CAD build for the part. Positions are in the model's coordinates, mm. Face numbers are marked on the shaded views. A direction names the side the tool comes from. Give positions to 0.01 mm unless a question says otherwise; leave off trailing zeros. Write each loop counter-clockwise with the first axis right and the second up, starting at its lowest first coordinate (ties: lowest second). Pieces come first, ordered by that corner, then holes. Notation, with made-up numbers: (-28, -33) - (1, -33) arc R17 ccw to (1, -15) - close; hole circle Ø11 at (-4.5, 60.5). An arc over 180 degrees is marked (long way). Answer as a JSON object with one key per item and string values.
from build123d import *

# Parameters (mm, degrees)
F1_DEPTH = 25.4
F2_SIZE  = 2.54
F3_SIZE  = 2.54
F4_T     = -1.27
F6_DEPTH = 38.1
F7_R     = 1.8028918562
F7_R_2   = 1.1064766703
F7_R_3   = 1.1353765366
F7_R_4   = 1.2323804773
F7_R_5   = 1.153275907
F8_DEPTH = 12.7


with BuildPart() as f1:
    # F0 (on Front) → F1 (new body)
    with BuildSketch(Plane.XZ):
        Polygon((44.08133775, 31.9471210241), (-47.1148937941, 31.9471210241), (-47.1148937941, -27.9655810446), (-25.1216236502, -27.9655810446), (-25.1216236502, -4.8347273842), (44.08133775, -4.8347273842), (44.08133775, 7.8682824969), (-25.1216236502, 7.8682824969), (-25.1216236502, 19.2441120744), (44.08133775, 19.2441120744), align=None)
    extrude(amount=F1_DEPTH)

    # F2
    f2_edges = [f1.edges().sort_by_distance(p)[0] for p in [
        (-1.516778, -25.4, 31.947121),
    ]]
    chamfer(f2_edges, length=F2_SIZE)

    # F3
    f3_edges = [f1.edges().sort_by_distance(p)[0] for p in [
        (44.081338, -25.4, 24.325617),
        (9.479857, -25.4, 19.244112),
        (-25.121624, -25.4, 13.556197),
        (9.479857, -25.4, 7.868282),
        (44.081338, -25.4, 1.516778),
        (9.479857, -25.4, -4.834727),
        (-25.121624, -25.4, -16.400154),
        (-36.118259, -25.4, -27.965581),
        (-47.114894, -25.4, 0.72077),
    ]]
    chamfer(f3_edges, length=F3_SIZE)

    # F4
    f4_openings = [f1.faces().sort_by_distance(p)[0] for p in [
        (-1.516778, 0, 30.855962),
    ]]
    offset(amount=F4_T, openings=f4_openings, kind=Kind.INTERSECTION)

    # F5 (on face) → F6 (cut, symmetric)
    with BuildSketch(Plane(origin=(0, 0, -4.8347273842), x_dir=(1, 0, 0), z_dir=(0, 0, -1))):
        with BuildLine():
            Line((44.08133775, 0), (44.08133775, 10.256701149))
            ThreePointArc((44.08133775, 10.256701149), (-1.820328138, 7.8273301251), (-47.1148937941, 0))
            Line((-47.1148937941, 0), (44.08133775, 0))
        make_face()
    extrude(amount=F6_DEPTH, both=True, mode=Mode.SUBTRACT)

    # F7 (on face) → F8 (join)
    with BuildSketch(Plane(origin=(0, -24.13, 0), x_dir=(-1, 0, 0), z_dir=(0, 1, 0))):
        with Locations((-36.7269202571, 25.4060197622)):
            Circle(F7_R)
        with Locations((-36.7269202571, 25.4060197622)):
            Circle(F7_R_2, mode=Mode.SUBTRACT)
        with Locations((0, 25.4060197622)):
            Circle(F7_R)
        with Locations((0, 25.4060197622)):
            Circle(F7_R_3, mode=Mode.SUBTRACT)
        with Locations((36.6482846439, 25.1216236502)):
            Circle(F7_R)
        with Locations((36.6482846439, 25.1216236502)):
            Circle(F7_R_4, mode=Mode.SUBTRACT)
        with Locations((36.6482846439, -20.2868953347)):
            Circle(F7_R)
        with Locations((36.6482846439, -20.2868953347)):
            Circle(F7_R_5, mode=Mode.SUBTRACT)
    extrude(amount=F8_DEPTH)


solid = f1.part
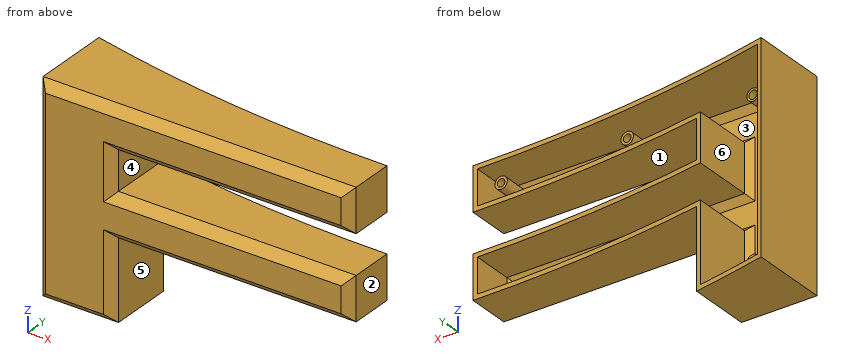
(1) Saw through at D-D, the plane x = -32.5. Give the cut face in (y, z), and give its area (3 significant figures).
Answer key:
{"outline": "(-25.4, -25.43) - (-22.86, -27.97) - (-3.13, -27.97) - (-3.13, -26.7) - (-22.33, -26.7) - (-24.13, -24.9) - (-24.13, 28.88) - (-22.33, 30.68) - (-3.13, 30.68) - (-3.13, 31.95) - (-22.86, 31.95) - (-25.4, 29.41) - close", "area": "126 mm²"}
(2) Saw through at A-A, the plane y = -20. State how many separate pieces and enclosed holes the cut face has, and give its area (3 significant figures).
Answer key:
{"separate pieces": "5", "enclosed holes": "5", "area": "577 mm²"}
(3) Saw through at B-B, the plane z = 2. Give the cut face in (x, y).
Answer key:
{"outline": "(-47.11, -22.86) - (-44.57, -25.4) - (41.54, -25.4) - (44.08, -22.86) - (44.08, -10.26) arc R388.97 cw to (42.81, -10.26) - (42.81, -22.33) - (41.02, -24.13) - (-44.05, -24.13) - (-45.84, -22.33) - (-45.84, -0.3) arc R388.97 cw to (-47.11, 0) - close"}
(4) Pull direction X, two halves, no side cores. Call the marked faces 1, 2 and 3: pulls with the +X half, pulls with the -X half, needs draft (parallel to the pull), parting line crosses it, or undercut.
Answer key:
{"face 1": "needs draft", "face 2": "pulls with the +X half", "face 3": "undercut"}
(5) Probe L1, parallel to Z at x = 0, y = -21; L2, parallel to Z at x = -21, y = -9; L3, parallel to X at y = -20.5, z = -6.5. List the from-to ranges inside material, lowest first. Write a range as [from, to].
Answer key:
{"L1": "z = [-4.83, -3.56], [6.6, 7.87], [19.24, 20.51], [23.6, 24.27], [26.54, 27.21], [30.68, 31.95]", "L2": "z = [-4.83, -3.56], [6.6, 7.87], [19.24, 20.51], [30.68, 31.95]", "L3": "x = [-47.11, -45.84], [-26.39, -25.12]"}
(6) Flat gauge pins, fed straight in: P1, Ø12, axis at x = 14, z = 11.5, coming from the -Y side; P2, Ø1, axis at x = -10, y = -7, coming from the -Z side; P3, Ø6, axis at x = -31.5, z = -19.5, coming from the +Y side. Where does each tip first touch, or does it go through?
Answer key:
{"P1": "stops at y = -25.23", "P2": "stops at z = -4.83", "P3": "stops at y = -24.13"}
(7) 3-axis set-ups, long thin cutter, end or side, ignore diameter. For the marked faces 4, 5 and 6: which of +Z, -Z, +X, -X, +Y, -Y reach the whole face in a straight line?
Answer key:
{"face 4": "+X, +Y, -Y", "face 5": "-Z, +X, +Y, -Y", "face 6": "+Y"}
